Input: dimensioned drawing with shaded views. Units: mm. Origin: part minimum x, y, z. A direction names the side the tool comes from. Give positions to 0.01 mm unless a question says otherwise; leave off trailing zeros. Order: outer loops, then holes, each group sorted by start corner. A loop starts at its lowest first (then second) coordinate and runs counter-clockwise, first axis right, second up.
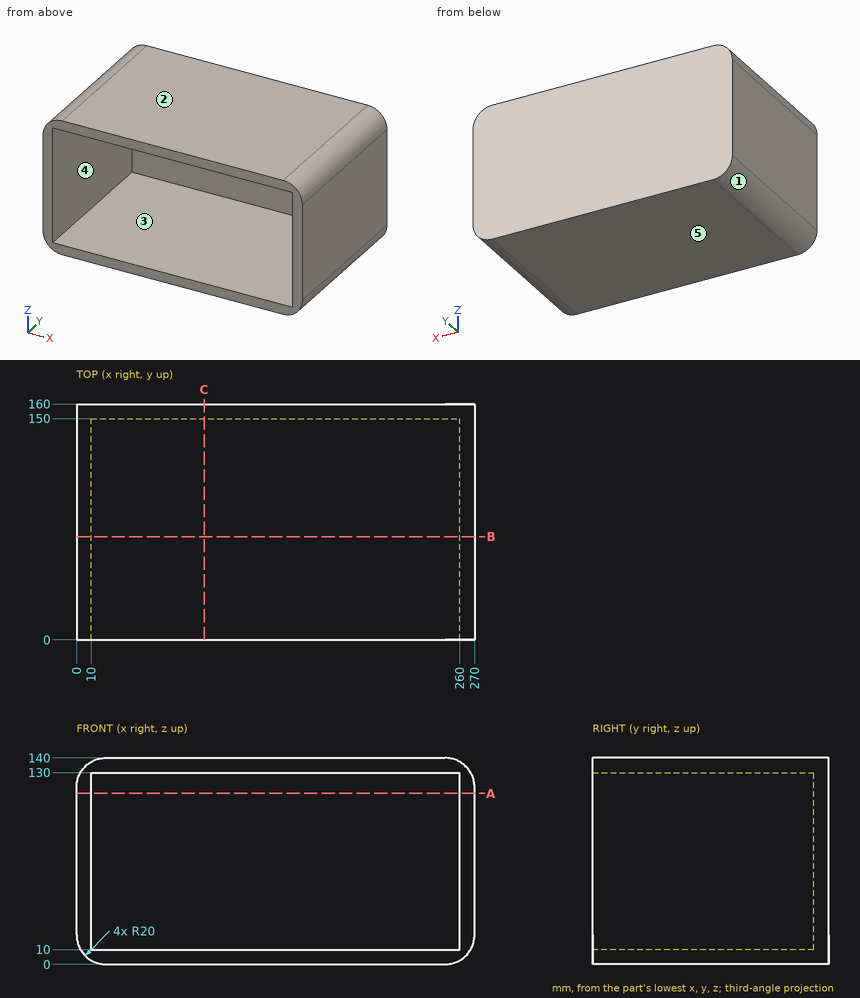
1) Line query: probe 1 along Z at (x, y) = (97.5, 68); probe 2 along X at (y, z) = (65.5, 81); probe 3 along Y at (x, z) = (184, 88.5). Output: solid intervals per line, ascending.
2) First-contact query: P1, Ø6, axis at y = 129, z = 72.5, coming from the -X side; P2, Ø1, axis at x = 80.5, z = 79.5, coming from the -Y side. Flat tips, straight axial feed; report the tip coordinate or a pass-through.
3) Pull-direction query (Z, two-part tool) for the marked faces 1, 2 and 3; classes: pulls with the +Z half, pulls with the -Z half, needs draft (parallel to the pull), parting line crosses it, or undercut.
4) Cut plane A-A (z = 116). Return the cut outline in (x, y).
5) Cut plane B-B (y = 70). Return the cut outline in (x, z).
6) Cut plane C-C (x = 86.5). Return the cut outline in (y, z), then the cut area to 3 significant figures.
7) Reachability of the marked faces 4 and 5 from +Z, -Z, +X, -X, +Y, -Y: full face, straight path, thin tool, end or side. Return the list, or none.
Geometry says:
1. probe 1: z = 0 to 10, 130 to 140
1. probe 2: x = 0 to 10, 260 to 270
1. probe 3: y = 150 to 160
2. P1: stops at x = 0
2. P2: stops at y = 150
3. face 1: pulls with the -Z half
3. face 2: pulls with the +Z half
3. face 3: undercut
4. outline: (0, 0) - (10, 0) - (10, 150) - (260, 150) - (260, 0) - (270, 0) - (270, 160) - (0, 160) - close
5. outline: (0, 20) arc R20 ccw to (20, 0) - (250, 0) arc R20 ccw to (270, 20) - (270, 120) arc R20 ccw to (250, 140) - (20, 140) arc R20 ccw to (0, 120) - close; hole (10, 10) - (260, 10) - (260, 130) - (10, 130) - close
6. outline: (0, 0) - (160, 0) - (160, 140) - (0, 140) - (0, 130) - (150, 130) - (150, 10) - (0, 10) - close
6. area: 4,400 mm2
7. face 4: -Y
7. face 5: -Z, +X, -X, +Y, -Y
